The listing builds one solid part. Answer for the finished solid, in the listing's coordinates (mm). A direction names the side the tool comes from. Round coordinates to 2 decimals unless told otherwise and drop trailing zeros. Loops run counter-clockwise (first coordinate to the right, second up) from the corner with the lowest first, then second, coordinate; pieces in that order, holes last. Notation, with made-up numbers: M 15.5,-35 L 64.5,-35 A36 ccw 64.5,0 Z; hole C 54.5,17.25 d9. An arc over 180 degrees is marked long. Put each result on its own line as item: value. Start each with the question number.
(1) Determine the mould class of faces 1 (the face through (4, 125, 112)), 2 (the face through (90, 476, 0)), 3 (the face through (90, 175, 0)) for opening direction Z: released by +Z, released by -Z, zero draft, split by the parting line, or undercut.
(2) Flat-ended cylindrical pins translate along their axes: P1, Ø5, axis at x = -2, y = 477, coming from the -Z side; P2, Ø11, axis at x = 92, y = 437.5, coming from the -Z side. Find the tip coordinate at first contact, or state that the pin passes through.
(3) Section B-B, the plane z = 38.5 is taken. Count the separate pieces of the cut face and the enclosed holes in it, then the cut area to 3 significant figures.
(4) Section C-C, the plane x = 27.5 is taken. Determine the outline of the cut face in (y, z), then the cut area to 3 significant figures.
(5) Section A-A, the plane y = 81.5 is taken. Determine the outline of the cut face in (x, z).
(6) Straight lines are drawn through the part: line 1 (Y direction, x = 85.5, z = 7.5); line 2 (X direction, y = 118, z = 35); line 3 (Z direction, x = 1, y = 80). For each, find the intervals that lie inside material, in ascending order.
(7) Which of the six approach directions +Z, -Z, +X, -X, +Y, -Y give full straight-line access (tool end or side, diameter ignored) to faces 4 (the face through (0, 476, 0)), 5 (the face through (44, -34, 102)), 6 (the face through (0, 55, 110))?
```python
from build123d import *

# Parameters (mm, degrees)
SKETCH1_W            = 10
SKETCH1_H            = 2
BOSS_EXTRUDE1_DEPTH  = 112
SKETCH2_W            = 10
SKETCH2_H            = 2
BOSS_EXTRUDE2_DEPTH  = 480
SKETCH3_W            = 10
SKETCH3_H            = 2
BOSS_EXTRUDE3_DEPTH  = 90
SKETCH4_W            = 10
SKETCH4_H            = 2
BOSS_EXTRUDE4_DEPTH  = 102
SKETCH5_W            = 10
SKETCH5_H            = 2
BOSS_EXTRUDE5_DEPTH  = 480
SKETCH6_W            = 10
SKETCH6_H            = 10
BOSS_EXTRUDE6_DEPTH  = 110
SKETCH7_W            = 10
SKETCH7_H            = 10
BOSS_EXTRUDE7_DEPTH  = 110
SKETCH8_W            = 10
SKETCH8_H            = 10
BOSS_EXTRUDE8_DEPTH  = 110
SKETCH9_W            = 10
SKETCH9_H            = 10
BOSS_EXTRUDE9_DEPTH  = 110
BOSS_EXTRUDE10_DEPTH = 70
SKETCH12_W           = 10
SKETCH12_H           = 2
BOSS_EXTRUDE11_DEPTH = 490


with BuildPart() as part:
    # Sketch1 → Boss-Extrude1 (new body)
    with BuildSketch(Plane.XY):
        Rectangle(SKETCH1_W, SKETCH1_H)
    extrude(amount=BOSS_EXTRUDE1_DEPTH)

    # Sketch2 → Boss-Extrude2 (add)
    with BuildSketch(Plane(origin=(0, 1, 0), x_dir=(1, 0, 0), z_dir=(0, 1, 0))):
        with Locations((0, -111)):
            Rectangle(SKETCH2_W, SKETCH2_H)
    extrude(amount=BOSS_EXTRUDE2_DEPTH)

    # Sketch3 → Boss-Extrude3 (add)
    with BuildSketch(Plane(origin=(5, 0, 0), x_dir=(0, 0, -1), z_dir=(1, 0, 0))):
        with Locations((-107, 0)):
            Rectangle(SKETCH3_W, SKETCH3_H)
    extrude(amount=BOSS_EXTRUDE3_DEPTH)

    # Sketch4 → Boss-Extrude4 (add)
    with BuildSketch(Plane(origin=(0, 0, 102), x_dir=(-1, 0, 0), z_dir=(0, 0, -1))):
        with Locations((-90, 0)):
            Rectangle(SKETCH4_W, SKETCH4_H)
    extrude(amount=BOSS_EXTRUDE4_DEPTH)

    # Sketch5 → Boss-Extrude5 (add)
    with BuildSketch(Plane(origin=(0, 1, 0), x_dir=(1, 0, 0), z_dir=(0, 1, 0))):
        with Locations((90, -111)):
            Rectangle(SKETCH5_W, SKETCH5_H)
    extrude(amount=BOSS_EXTRUDE5_DEPTH)

    # Sketch6 → Boss-Extrude6 (add)
    with BuildSketch(Plane(origin=(0, 0, 110), x_dir=(-1, 0, 0), z_dir=(0, 0, -1))):
        with Locations((-90, 116)):
            Rectangle(SKETCH6_W, SKETCH6_H)
        with Locations((0, 116)):
            Rectangle(SKETCH6_W, SKETCH6_H)
    extrude(amount=BOSS_EXTRUDE6_DEPTH)

    # Sketch7 → Boss-Extrude7 (add)
    with BuildSketch(Plane(origin=(0, 0, 110), x_dir=(-1, 0, 0), z_dir=(0, 0, -1))):
        with Locations((-90, 236)):
            Rectangle(SKETCH7_W, SKETCH7_H)
        with Locations((0, 236)):
            Rectangle(SKETCH7_W, SKETCH7_H)
    extrude(amount=BOSS_EXTRUDE7_DEPTH)

    # Sketch8 → Boss-Extrude8 (add)
    with BuildSketch(Plane(origin=(0, 0, 110), x_dir=(-1, 0, 0), z_dir=(0, 0, -1))):
        with Locations((-90, 356)):
            Rectangle(SKETCH8_W, SKETCH8_H)
        with Locations((0, 356)):
            Rectangle(SKETCH8_W, SKETCH8_H)
    extrude(amount=BOSS_EXTRUDE8_DEPTH)

    # Sketch9 → Boss-Extrude9 (add)
    with BuildSketch(Plane(origin=(0, 0, 110), x_dir=(-1, 0, 0), z_dir=(0, 0, -1))):
        with Locations((-90, 476)):
            Rectangle(SKETCH9_W, SKETCH9_H)
        with Locations((0, 476)):
            Rectangle(SKETCH9_W, SKETCH9_H)
    extrude(amount=BOSS_EXTRUDE9_DEPTH)

    # Sketch11 → Boss-Extrude10 (add)
    with BuildSketch(Plane.XZ.offset(1)):
        Polygon((-5, 112), (-5, 0), (5, 0), (5, 102), (85, 102), (85, 0), (95, 0), (95, 112), align=None)
    extrude(amount=BOSS_EXTRUDE10_DEPTH)

    # Sketch12 → Boss-Extrude11 (add)
    with BuildSketch(Plane.XZ.offset(71)):
        with Locations((90, -1)):
            Rectangle(SKETCH12_W, SKETCH12_H)
        with Locations((0, -1)):
            Rectangle(SKETCH12_W, SKETCH12_H)
    extrude(amount=-BOSS_EXTRUDE11_DEPTH)


solid = part.part
```
Recorded:
1. face 1: released by +Z
1. face 2: released by -Z
1. face 3: undercut
2. P1: stops at z = 0
2. P2: stops at z = 110
3. separate pieces: 10
3. enclosed holes: 0
3. area: 2,240 mm²
4. outline: M -71,102 L 1,102 L 1,112 L -71,112 Z
4. area: 720 mm²
5. outline: M -5,-2 L 5,-2 L 5,0 L -5,0 Z; M -5,110 L 5,110 L 5,112 L -5,112 Z; M 85,-2 L 95,-2 L 95,0 L 85,0 Z; M 85,110 L 95,110 L 95,112 L 85,112 Z
6. line 1: y = -71 to 1, 111 to 121, 231 to 241, 351 to 361, 471 to 481
6. line 2: x = -5 to 5, 85 to 95
6. line 3: z = -2 to 0, 110 to 112
7. face 4: -Z, +X, -X, +Y
7. face 5: -Z, +Y, -Y
7. face 6: +X, -X
